Work out the finished part from the listing and answer in its coordinate system (mm). A direction names the side the tool comes from. Coordinates: 2 decimals unless noted, no trailing zeros. Order: outer loops, then holes, each group sorted by start corner. A loop starts at its lowest first (then second) coordinate and runs counter-clockwise, first axis right, second up. Notation, with made-up numbers: M -11.75,17.25 L -2.75,17.25 A27 cw -2.75,47.25 Z; hole C 1,75 d3. An arc over 180 degrees is marked long. Write item = value, one per line. Start each with the question number.
Q1. A tool of negligible diameter and unlimited length cuts with its end or side. For faces 4 (the cylindrical face through (16.279, -119.143, 70.885)), 5 (the cylindrical face through (50.62, -125.2, 68.98)), from which of +Z, -Z, +X, -X, +Y, -Y can it reach the whole face along a straight path? Write none if from no direction.
Q2. Determine the mould class of faces 1 (the flat face through (63.5, -127.6, 66.7)), 2 (the cylindrical face through (32.194, -129.236, 67.251)), 3 (the conical face through (37.853, -125.706, 71.98)) for opening direction Z: released by +Z, released by -Z, zero draft, split by the parting line, or undercut.
Q3. Straight lines are drawn through the part: line 1 along Z through (x, y) = (32.5, -129); line 2 along X through (y, z) = (-125, 70); line 3 along Z through (x, y) = (43.5, -128.75). For each, find the intervals that lie inside material, in ascending order.
Q4. Find section A-A on x = 15.5. Give the vertices of the cut face in (y, z) (3 decimals), and give its area (3 significant figures).
Q5. Each of these flat-tipped pins is pushed along its axis until it touches: P1, Ø1, axis at x = 34.5, z = 75, coming from the -Y side; P2, Ø10, axis at x = 48, y = -122.5, coming from the -Z side; P3, Ø4, axis at y = -128.23, z = 68.02, coming from the +X side; P4, Ø1.5, axis at x = 32, z = 61.5, coming from the +Y side. Where does it stop, or does it pass through?
Q6. Find section B-B on x = 44.5. Give the vertices of the cut face in (y, z) (3 decimals).
```python
from build123d import *

# Parameters (mm, degrees)
F0_R     = 9.525
F1_DEPTH = 38.1
F2_SIZE  = 5.08
F3_R     = 3.175
F4_DEPTH = 25.4
F5_R     = 1.27
F6_DEPTH = 189.484


with BuildPart() as f1:
    # F0 (on Right) → F1 (new body)
    with BuildSketch(Plane.YZ):
        with Locations((-128.22786, 68.024091)):
            Circle(F0_R)
    extrude(amount=F1_DEPTH)

    # F2
    f2_edges = [f1.edges().sort_by_distance(p)[0] for p in [
        (38.1, -137.75286, 68.024091),
    ]]
    chamfer(f2_edges, length=F2_SIZE)

    # F3 (on face) → F4 (join)
    with BuildSketch(Plane.YZ.offset(38.1)):
        with Locations((-128.22786, 68.024091)):
            Circle(F3_R)
    extrude(amount=F4_DEPTH)

    # F5 (on face) → F6 (cut)
    with BuildSketch(Plane.YZ.offset(63.5)):
        with Locations((-128.22786, 68.024091)):
            Circle(F5_R)
    extrude(amount=-F6_DEPTH, mode=Mode.SUBTRACT)


solid = f1.part
```
Findings below:
q1.face_4 = +X, -X
q1.face_5 = +X
q2.face_1 = zero draft
q2.face_2 = undercut
q2.face_3 = split by the parting line
q3.line_1 = 58.53 to 67.02, 69.03 to 77.52
q3.line_2 = 0 to 38.1
q3.line_3 = 64.89 to 66.87, 69.18 to 71.16
q4.outline = C -128.228,68.024 d19.05; hole C -128.228,68.024 d2.54
q4.area = 280 mm^2
q5.P1 = -133.4
q5.P2 = 64.93
q5.P3 = 63.5
q5.P4 = -120.65
q6.outline = C -128.228,68.024 d6.35; hole C -128.228,68.024 d2.54
